```python
from build123d import *

# Parameters (mm, degrees)
SKETCH1_R             = 30
SKETCH1_R_2           = 25
BOSS_EXTRUDE1_DEPTH   = 40
SKETCH4_R             = 15
SKETCH4_R_2           = 10
BOSS_EXTRUDE2_DEPTH   = 20
BOSS_EXTRUDE2_2_DEPTH = 20
BOSS_EXTRUDE3_START   = 5
BOSS_EXTRUDE3_DEPTH   = 5


with BuildPart() as part:
    # Sketch1 → Boss-Extrude1 (new body)
    with BuildSketch(Plane(origin=(0, 0, 0), x_dir=(1, 0, 0), z_dir=(0, 1, 0))):
        with Locations(Location((0, 0, 0), (0, 0, 270))):
            Circle(SKETCH1_R)
        with Locations(Location((0, 0, 0), (0, 0, 270))):
            Circle(SKETCH1_R_2, mode=Mode.SUBTRACT)
    extrude(amount=BOSS_EXTRUDE1_DEPTH)


with BuildPart() as body_2:
    # Sketch4 → Boss-Extrude2 (new, symmetric)
    with BuildSketch(Plane.XY):
        with Locations((-110, 0)):
            Circle(SKETCH4_R)
        with Locations((-110, 0)):
            Circle(SKETCH4_R_2, mode=Mode.SUBTRACT)
    extrude(amount=BOSS_EXTRUDE2_DEPTH, both=True)



with BuildPart() as body_3:
    # Sketch4 → Boss-Extrude2 2 (new, symmetric)
    with BuildSketch(Plane.XY):
        with Locations(Location((110, 0, 0), (0, 0, 180))):
            Circle(SKETCH4_R)
        with Locations(Location((110, 0, 0), (0, 0, 180))):
            Circle(SKETCH4_R_2, mode=Mode.SUBTRACT)
    extrude(amount=BOSS_EXTRUDE2_2_DEPTH, both=True)


with BuildPart() as body_2_1:
    add(body_2.part)

    add(body_3.part)  # Boss-Extrude3 merges body 3
    # Sketch5 → Boss-Extrude3 (add)
    with BuildSketch(Plane.XY.offset(BOSS_EXTRUDE3_START)):
        with BuildLine():
            Line((-114.363197033, 14.351394066), (-30, 40))
            Line((-30, 40), (-25, 40))
            Line((-25, 40), (-25, 0))
            Line((-25, 0), (-30, 0))
            Line((-30, 0), (-107.1875, -14.733969043))
            ThreePointArc((-107.1875, -14.733969043), (-95.436664114, 3.59294418), (-114.363197033, 14.351394066))
        make_face()
        with BuildLine():
            Line((30, 0), (107.1875, -14.733969043))
            ThreePointArc((107.1875, -14.733969043), (95.436664114, 3.59294418), (114.363197033, 14.351394066))
            Line((114.363197033, 14.351394066), (30, 40))
            Line((30, 40), (25, 40))
            Line((25, 40), (25, 0))
            Line((25, 0), (30, 0))
        make_face()
    boss_extrude3 = extrude(amount=BOSS_EXTRUDE3_DEPTH)


with BuildPart() as part_1:
    add(part.part)

    add(body_2_1.part)  # Mirror2 merges body 2
    # Mirror2: Boss-Extrude3 across plane
    add(boss_extrude3.mirror(Plane.XY))


solid = part_1.part
```
Here's how the part is built. I have some questions about the finished solid (model axes, mm). A direction names the side the tool comes from. Give positions to 0.01 mm unless a question says otherwise; leave off trailing zeros. Write each loop counter-clockwise with the first axis right and the second up, starting at its lowest first coordinate (ties: lowest second). Pieces come first, ordered by that corner, then holes.
(1) Thinking about a two-plate mould opening in X: for faces 6 (the face through (-62, 13, -5)), 7 (the face through (-100, -3, 20)), 8 (the face through (-72.772, 26.996, -7.465)), which applies, pulls with the +X half, pulls with the -X half, needs draft (parallel to the pull), parting line crosses it, or undercut?
Output values:
face 6: undercut
face 7: needs draft
face 8: pulls with the -X half
(2) If I drill on L1, parallel to Y at x = -110, z = 4.5; L2, parallel to Z at x = 79, y = 16.5; L3, parallel to X at y = 3, z = 9, over which ranges is the centre line in solid material (lowest first)?
Output values:
L1: y = -15 to -10, 10 to 15
L2: z = -10 to -5, 5 to 10
L3: x = -124.7 to -119.54, -100.46 to -23.32, 23.32 to 100.46, 119.54 to 124.7
(3) On a 3-axis mill with a long thin cutter (end or side, diameter ignored), from which of +Z, -Z, +X, -X, +Y, -Y can I reach the whole of each face in a straight line? I mean faces 1 (the face through (0.517, 19.72, -29.996)), 2 (the face through (121.056, -10.138, 0.28)), 3 (the face through (-120, 0, 0)), 4 (the face through (100, 3, 20)), 5 (the face through (68.053, -7.264, -7.465)). Say none if no direction works.
Output values:
face 1: -Z, +Y, -Y
face 2: none
face 3: +Z, -Z
face 4: +Z, +X, +Y, -Y
face 5: +Z, -Z, -Y
(4) Imagine slicing it at B-B, the plane x = 0. Write out the boundary of the cut face in (y, z), and give its area (3 significant figures).
Output values:
outline: (0, -30) - (40, -30) - (40, -25) - (0, -25) - close; (0, 25) - (40, 25) - (40, 30) - (0, 30) - close
area: 400 mm2
(5) Imagine slicing it at D-D, the plane x = 110. Write out the boundary of the cut face in (y, z), and give its area (3 significant figures).
Output values:
outline: (-15, -20) - (-10, -20) - (-10, 20) - (-15, 20) - close; (10, -20) - (15, -20) - (15, -10) - (15.68, -10) - (15.68, -5) - (15, -5) - (15, 5) - (15.68, 5) - (15.68, 10) - (15, 10) - (15, 20) - (10, 20) - close
area: 407 mm2
(6) Will these pins go through, and if not, where does the flat tip stop? pin 1 (15 mm diameter, centred on x = 107, y = -1, fed in from +Z); pin 2 (10 mm diameter, centred on x = -46.5, z = 10.5, fed in from -Y); pin 3 (18 mm diameter, centred on x = -8.5, z = -4.5, fed in from -Y); pin 4 (1.5 mm diameter, centred on x = 23, y = 4.5, fed in from +Z).
Output values:
pin 1: stops at z = 20
pin 2: stops at y = -4.1
pin 3: passes through
pin 4: stops at z = 20.12
(7) Imagine slicing it at C-C, the plane y = 21.5. Write out the boundary of the cut face in (x, z).
Output values:
outline: (-90.85, -10) - (-28.28, -10) arc R30 ccw to (28.28, -10) - (90.85, -10) - (90.85, -5) - (29.58, -5) arc R30 ccw to (29.58, 5) - (90.85, 5) - (90.85, 10) - (28.28, 10) arc R30 ccw to (-28.28, 10) - (-90.85, 10) - (-90.85, 5) - (-29.58, 5) arc R30 ccw to (-29.58, -5) - (-90.85, -5) - close; hole circle Ø50 at (0, 0)
(8) Imagine slicing it at A-A, the plane z = 0. Write out the boundary of the cut face in (x, y).
Output values:
outline: circle Ø30 at (-110, 0); (-30, 0) - (-25, 0) - (-25, 40) - (-30, 40) - close; (25, 0) - (30, 0) - (30, 40) - (25, 40) - close; circle Ø30 at (110, 0); hole circle Ø20 at (-110, 0); hole circle Ø20 at (110, 0)
